```python
from build123d import *

# Parameters (mm, degrees)
CORTAR_EXTRUIR1_DEPTH = 2
CHAFL_N1_SIZE         = 0.5
REDONDEO1_R           = 0.5


with BuildPart() as part:
    # Croquis1 → Revolución1 (revolve)
    with BuildSketch(Plane.XY):
        Polygon((0, 0), (2.25, 0), (2.25, -2.5), (1.25, -2.5), (1.25, -12.5), (0, -12.5), align=None)
    revolve(axis=Axis((0, 0, 0), (0, -1, 0)))

    # Croquis2 → Cortar-Extruir1 (cut)
    with BuildSketch(Plane(origin=(0, 0, 0), x_dir=(1, 0, 0), z_dir=(0, 1, 0))):
        Polygon((1, 0.577350269), (0, 1.154700538), (-1, 0.577350269), (-1, -0.577350269), (0, -1.154700538), (1, -0.577350269), align=None)
    extrude(amount=-CORTAR_EXTRUIR1_DEPTH, mode=Mode.SUBTRACT)

    # Chaflán1
    chafl_n1_edges = [part.edges().sort_by_distance(p)[0] for p in [
        (-1.25, -12.5, 0),
    ]]
    chamfer(chafl_n1_edges, length=CHAFL_N1_SIZE)

    # Redondeo1
    redondeo1_edges = [part.edges().sort_by_distance(p)[0] for p in [
        (-2.25, 0, 0),
    ]]
    fillet(redondeo1_edges, radius=REDONDEO1_R)


solid = part.part
```
The model under review builds one solid part; all positions refer to its coordinate system, in mm. A direction names the side the tool comes from. Round coordinates to 2 decimals unless told otherwise and drop trailing zeros. Write each loop counter-clockwise with the first axis right and the second up, starting at its lowest first coordinate (ties: lowest second). Pieces come first, ordered by that corner, then holes. Notation, with made-up numbers: (59.5, 74.5) - (72.5, 74.5) arc R37 cw to (72.5, 112.5) - close; hole circle Ø5 at (72, 12). An arc over 180 degrees is marked (long way). Use one line per item in the form item = value.
Q1. For line 1 (Y direction, x = 1.35, z = 0.55); line 2 (X direction, y = -8.5, z = 1); line 3 (Z direction, x = 0, y = -10.5), list the stretches that pass through material, from the lowest coordinate up. Write a range as [from, to].
Answer key:
line_1 = [-2.5, 0]
line_2 = [-0.75, 0.75]
line_3 = [-1.25, 1.25]
Q2. Insertion check: pin 1 Ø1.5 at (x, y) = (-0.5, -7.5) entering from -Z; pin 2 Ø0.6 at (x, z) = (0, 0) entering from +Y. Each pin has a flat end and moves straight along its axis. Give the tip position at first contact, or say it passes through.
Answer key:
pin_1 = -1.25
pin_2 = -2
Q3. Draft analysis for pull direction Z (two halves, no side actions). For faces 4 (the cylindrical face through (-0.29, -1.51, 2.23)), 5 (the flat face through (-0.51, -0.99, 0.86)), 6 (the flat face through (1, -2.5, -1)), state which applies: +Z half, -Z half, draft (parallel to the pull), parting line (faces both ways), or undercut.
Answer key:
face_4 = parting line
face_5 = undercut
face_6 = draft
Q4. Tool access review of faces 1 (the cylindrical face through (-0.27, -7.32, -1.22)), 2 (the flat face through (0, -12.5, 0)), 3 (the flat face through (0.49, -0.99, 0.87)): name each direction out of +Z, -Z, +X, -X, +Y, -Y from which nothing blocks a thin tool from reaching the whole face with its end or side.
Answer key:
face_1 = -Y
face_2 = +Z, -Z, +X, -X, -Y
face_3 = +Y
Q5. Consider section A-A (z = 0). State the section outline as (x, y) points, and give its area (3 significant figures).
Answer key:
outline = (-2.25, -2.5) - (-1.25, -2.5) - (-1.25, -12) - (-0.75, -12.5) - (0.75, -12.5) - (1.25, -12) - (1.25, -2.5) - (2.25, -2.5) - (2.25, -0.5) arc R0.5 ccw to (1.75, 0) - (1, 0) - (1, -2) - (-1, -2) - (-1, 0) - (-1.75, 0) arc R0.5 ccw to (-2.25, -0.5) - close
area = 31.9 mm2
Q6. Consider section B-B (y = -3). State the section outline as (x, z) points, and give its area (3 significant figures).
Answer key:
outline = circle Ø2.5 at (0, 0)
area = 4.91 mm2
